Build history of the part. All positions in model axes, mm. Give positions to 0.01 mm unless a question says otherwise; leave off trailing zeros. Write each loop counter-clockwise with the first axis right and the second up, starting at its lowest first coordinate (ties: lowest second). Pieces come first, ordered by that corner, then holes. Notation, with made-up numbers: (63, -6.5) -> (91, -6.5) arc R27 cw to (91, 14.5) -> close; hole circle Ø1 at (70.5, 5.5). An arc over 180 degrees is marked (long way). Put each result on its own line as item: value.
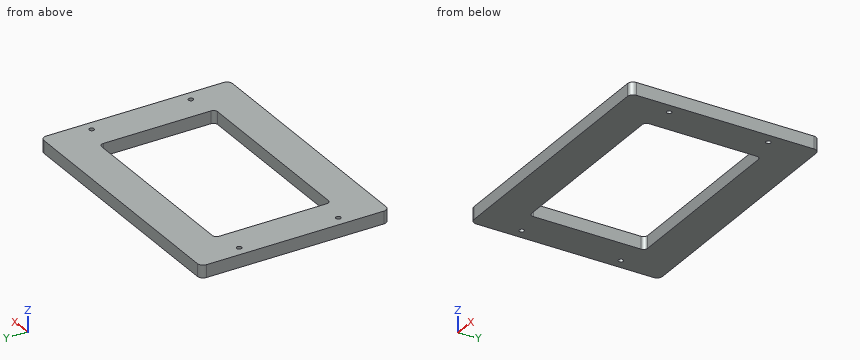
from build123d import *

# Parameters (mm, degrees)
SKETCH_W        = 187
SKETCH_H        = 135
PAD_DEPTH       = 9
SKETCH001_R     = 1.75
POCKET_DEPTH    = 9.001
FILLET_R        = 4
SKETCH002_W     = 135
SKETCH002_H     = 83
POCKET001_DEPTH = 9.001
FILLET001_R     = 3


with BuildPart() as part:
    # Sketch → Pad (new body)
    with BuildSketch(Plane.XY):
        Rectangle(SKETCH_W, SKETCH_H)
    extrude(amount=PAD_DEPTH)

    # Sketch001 (on Face6 of Pad) → Pocket (cut, through all)
    with BuildSketch(Plane.XY.offset(9)):
        with Locations((-86, 35.5)):
            Circle(SKETCH001_R)
        with Locations((86, 35.5)):
            Circle(SKETCH001_R)
        with Locations((-86, -35.5)):
            Circle(SKETCH001_R)
        with Locations((86, -35.5)):
            Circle(SKETCH001_R)
    extrude(amount=-POCKET_DEPTH, mode=Mode.SUBTRACT)

    # Fillet
    fillet_edges = [part.edges().sort_by_distance(p)[0] for p in [
        (-93.5, 67.5, 4.5),
        (-93.5, -67.5, 4.5),
        (93.5, -67.5, 4.5),
        (93.5, 67.5, 4.5),
    ]]
    fillet(fillet_edges, radius=FILLET_R)

    # Sketch002 (on Face5 of Fillet) → Pocket001 (cut, through all)
    with BuildSketch(Plane.XY.offset(9)):
        Rectangle(SKETCH002_W, SKETCH002_H)
    extrude(amount=-POCKET001_DEPTH, mode=Mode.SUBTRACT)

    # Fillet001
    fillet001_edges = [part.edges().sort_by_distance(p)[0] for p in [
        (-67.5, 41.5, 4.5),
        (-67.5, -41.5, 4.5),
        (67.5, -41.5, 4.5),
        (67.5, 41.5, 4.5),
    ]]
    fillet(fillet001_edges, radius=FILLET001_R)


solid = part.part
1) Wall check: L1, parallel to Y at x = 86, z = 3; L2, parallel to Y at x = -2.5, z = 3; L3, parallel to X at y = 30, z = 3.5. Give the ranges that are in metal, low to high.
Filled sheet:
L1: -67.5 to -37.25, -33.75 to 33.75, 37.25 to 67.5
L2: -67.5 to -41.5, 41.5 to 67.5
L3: -93.5 to -67.5, 67.5 to 93.5
2) Slice it at A-A (y = -4). Write the cut outline in (x, z), plus the area to 3 significant figures.
Filled sheet:
outline: (-93.5, 0) -> (-67.5, 0) -> (-67.5, 9) -> (-93.5, 9) -> close; (67.5, 0) -> (93.5, 0) -> (93.5, 9) -> (67.5, 9) -> close
area: 468 mm2
3) Slice it at C-C (z = 1.75). Write the cut outline in (x, y).
Filled sheet:
outline: (-93.5, -63.5) arc R4 ccw to (-89.5, -67.5) -> (89.5, -67.5) arc R4 ccw to (93.5, -63.5) -> (93.5, 63.5) arc R4 ccw to (89.5, 67.5) -> (-89.5, 67.5) arc R4 ccw to (-93.5, 63.5) -> close; hole circle Ø3.5 at (-86, -35.5); hole circle Ø3.5 at (-86, 35.5); hole (-67.5, -38.5) arc R3 ccw to (-64.5, -41.5) -> (64.5, -41.5) arc R3 ccw to (67.5, -38.5) -> (67.5, 38.5) arc R3 ccw to (64.5, 41.5) -> (-64.5, 41.5) arc R3 ccw to (-67.5, 38.5) -> close; hole circle Ø3.5 at (86, -35.5); hole circle Ø3.5 at (86, 35.5)
4) Slice it at B-B (x = 53.5). Write the cut outline in (y, z), plus the area to 3 significant figures.
Filled sheet:
outline: (-67.5, 0) -> (-41.5, 0) -> (-41.5, 9) -> (-67.5, 9) -> close; (41.5, 0) -> (67.5, 0) -> (67.5, 9) -> (41.5, 9) -> close
area: 468 mm2
5) Pin check, flat tips, straight feed: pin 1 (10 mm diameter, centred on x = 67.5, y = 44.5, fed in from -Z); pin 2 (2 mm diameter, centred on x = -86, y = 35.5, fed in from +Z). Stop position of each tip, or through.
Filled sheet:
pin 1: z = 0
pin 2: through
